Autodesk Inventor part; units mm, degrees
ref_plane "YZ Plane" through (0, 0, 0) normal (1, 0, 0) x (0, 1, 0)
ref_plane "XZ Plane" through (0, 0, 0) normal (0, 1, 0) x (-1, 0, 0)
ref_plane "XY Plane" through (0, 0, 0) normal (0, 0, 1) x (1, 0, 0)
sketch "Sketch1" plane through (0, 0, 0) normal (0, 0, 1) x (1, 0, 0)
  line L0 (-2.5, 0) -> (-9, 0)
  ellipse E0 centre (-4.792, 0) end of major axis (-9, 0) minor radius 2.5316 (-6.3785, 2.3447) -> (-6.3785, -2.3447) ccw
  arc A0 (-6.3785, -2.3447) -> (-6.3785, 2.3447) centre (0, 0) ccw
  line L1 (-6.3785, 2.3447) -> (-6.225, 2.482)
  circle A1 centre (0, 0) radius 2.5
  dimension "d2" = 6.5
  dimension "d4" = 5
extrude "Extrusion1" add sketch "Sketch1" along normal blind 7
sketch "Sketch2" plane through (0, 0, 7) normal (0, 0, 1) x (1, 0, 0)
  circle A0 centre (0, 0) radius 2.5
  arc A1 (-6.3785, -2.3447) -> (-6.3785, 2.3447) centre (0, 0) ccw
  line L0 (4.7343, 0) -> (2.3671, -4.1)
  line L1 (2.3671, -4.1) -> (-2.3671, -4.1)
  line L2 (-2.3671, -4.1) -> (-4.7343, 0)
  line L3 (-4.7343, 0) -> (-2.3671, 4.1)
  line L4 (-2.3671, 4.1) -> (2.3671, 4.1)
  line L5 (2.3671, 4.1) -> (4.7343, 0)
  dimension "d7" = 8.2
extrude "Extrusion2" cut sketch "Sketch2" against normal blind 4
properties part number "cam4.0"
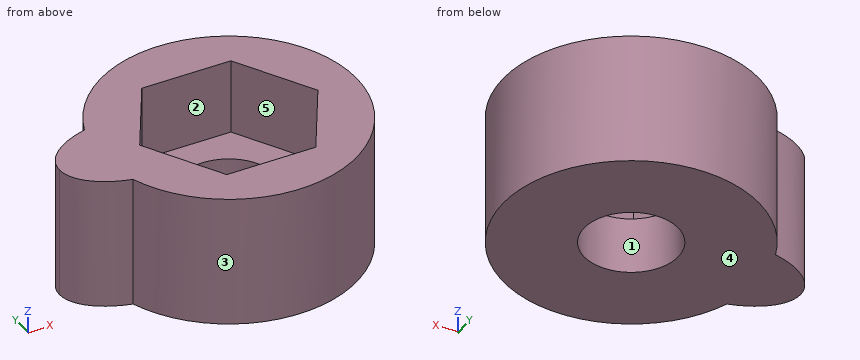
Here's how the part is built. I have some questions about the finished solid (model axes, mm). Face numbers are marked on the shaded views. A direction names the side the tool comes from. Round coordinates to 2 decimals unless told otherwise and drop trailing zeros. Order: outer loops, then holes, each group sorted by start corner. A loop starts at its lowest first (then second) coordinate and runs counter-clockwise, first axis right, second up. Notation, with made-up numbers: M 48.5,-13 L 76.5,-13 A24 cw 76.5,25 Z; hole C -38,77 d9. An arc over 180 degrees is marked long. Answer in a Markdown table with one row per item.
Item 1: Imagine slicing it at D-D, the plane y = -4.5. Write out the boundary of the cut face in (x, z), and give its area (3 significant figures).
A:
| item | result |
|---|---|
| outline | M -5.09,0 L 5.09,0 L 5.09,7 L -5.09,7 Z |
| area | 71.3 mm2 |
Item 2: Imagine slicing it at C-C, the plane x = -3.5. Write out the boundary of the cut face in (y, z).
A:
| item | result |
|---|---|
| outline | M -5.83,0 L 5.83,0 L 5.83,7 L 2.14,7 L 2.14,3 L -2.14,3 L -2.14,7 L -5.83,7 Z |
Item 3: Thinking about a two-plate mould opening in Y: for the marked faces 3, 4 and 5, which applies, +Y half, -Y half, draft (parallel to the pull), parting line (faces both ways), or undercut?
A:
| item | result |
|---|---|
| face 3 | parting line |
| face 4 | draft |
| face 5 | undercut |
Item 4: I'm going to push flat-ended pins straight in: pin 1 (4.5 mm diameter, centred on x = 0, y = 0, fed in from -Z); pin 2 (1.5 mm diameter, centred on x = -5, z = 3, fed in from -Y); pin 3 (1 mm diameter, centred on x = -6.5, z = 5, fed in from -Y). Where does each tip first touch, or does it pass through?
A:
| item | result |
|---|---|
| pin 1 | passes through |
| pin 2 | stops at y = -5.3 |
| pin 3 | stops at y = -3.19 |
Item 5: For the marked faces 1 and 2, which set-ups out of +Z, -Z, +X, -X, +Y, -Y let a thin tool reach every point of the face, with its end or its side?
A:
| item | result |
|---|---|
| face 1 | +Z, -Z |
| face 2 | +Z |
Item 6: If I drill on L1, parallel to Y at x = 0, z = 0.75; L2, parallel to Y at x = 4, z = 3.25; L3, parallel to X at y = 0.5, z = 2.5, over which ranges is the centre line in solid material (lowest first)? Write a range as from..to.
A:
| item | result |
|---|---|
| L1 | y = -6.8..-2.5, 2.5..6.8 |
| L2 | y = -5.49..-1.27, 1.27..5.49 |
| L3 | x = -8.92..-2.45, 2.45..6.78 |
Item 7: Imagine slicing it at A-A, the plane x = 0. Write out the boundary of the cut face in (y, z).
A:
| item | result |
|---|---|
| outline | M -6.8,0 L -2.5,0 L -2.5,3 L -4.1,3 L -4.1,7 L -6.8,7 Z; M 2.5,0 L 6.8,0 L 6.8,7 L 4.1,7 L 4.1,3 L 2.5,3 Z |
Item 8: Imagine slicing it at B-B, the plane y = -3. Write out the boundary of the cut face in (x, z).
A:
| item | result |
|---|---|
| outline | M -6.1,0 L 6.1,0 L 6.1,7 L 3,7 L 3,3 L -3,3 L -3,7 L -6.1,7 Z |
